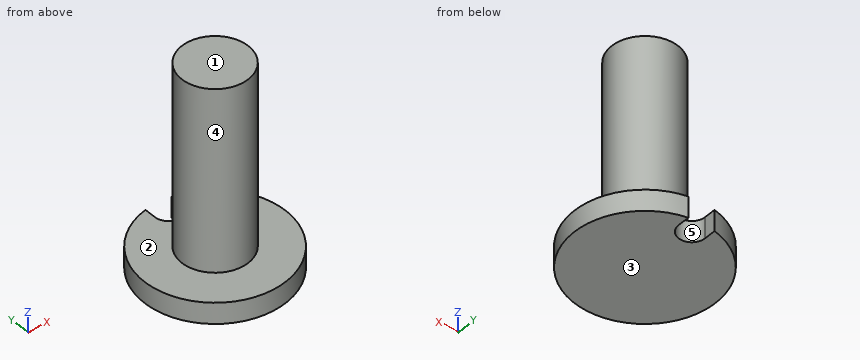
Autodesk Inventor part; units mm, degrees
ref_plane "YZ Plane" through (0, 0, 0) normal (1, 0, 0) x (0, 1, 0)
ref_plane "XZ Plane" through (0, 0, 0) normal (0, 1, 0) x (-1, 0, 0)
ref_plane "XY Plane" through (0, 0, 0) normal (0, 0, 1) x (1, 0, 0)
sketch "Sketch1" plane through (0, 0, 0) normal (0, 0, 1) x (1, 0, 0)
  circle A0 centre (0, 0) radius 8.509
  dimension "d0" = 17.018
extrude "Extrusion1" add sketch "Sketch1" along normal blind 2.54
sketch "Sketch3" plane through (0, 0, 0) normal (0, 0, -1) x (-1, 0, 0)
  line L0 (0, 0) -> (0, 6.9342)
  circle A0 centre (0, 6.9342) radius 1.5875
  line L1 (-1.5875, 6.9342) -> (-1.5875, 8.3596)
  circle A1 centre (0, 0) radius 8.509
  line L2 (1.5875, 6.9342) -> (1.5875, 8.3596)
  dimension "d6" = 6.9342
  dimension "d7" = 3.175
extrude "Extrusion3" cut sketch "Sketch3" against normal through all contours A0 A1 | A0 A1 L2 | A0 L1 A1 picked at (-0.1424, 6.414)
sketch "Sketch2" plane through (0, 0, 2.54) normal (0, 0, 1) x (1, 0, 0)
  circle A0 centre (0, 0) radius 8.509
  circle A1 centre (0, 0) radius 4.0005
  dimension "d3" = 8.001
extrude "Extrusion2" add sketch "Sketch2" along normal blind 21.971 contours A1
properties part number "pulley shaft"
Check sheet for the modelled part. Datum: model origin and axes. Units: mm. Face numbers are marked on the shaded views. A direction names the side the tool comes from. Give positions to 0.01 mm unless a question says otherwise; leave off trailing zeros. Write each loop counter-clockwise with the first axis right and the second up, starting at its lowest first coordinate (ties: lowest second). Pieces come first, ordered by that corner, then holes. Notation, with made-up numbers: (83.25, 64) -> (111.25, 64) arc R10 cw to (111.25, 73) -> close; hole circle Ø5 at (35, -3.75). An arc over 180 degrees is marked (long way). Use one line per item in the form item = value. Start each with the question number.
1. Go/stop test with flat-tipped pins: P1, Ø6, axis at y = 0.5, z = 19.5, coming from the +X side; P2, Ø5, axis at x = 0.5, z = 9.5, coming from the -Y side; P3, Ø4, axis at y = 5, z = 15, coming from the -X side. Record where each tip stops, or that it passes through.
2. Access from +Z, -Z, +X, -X, +Y, -Y to the whole of each face (thin tool, end or side, straight path). Record for the marked faces 1 and 2.
3. Section check D-D (x = -7). Record the cut outline in (y, z), and give its area (3 significant figures).
4. Section check A-A (x = 0). Record the cut outline in (y, z).
5. Thickness scan on line 1 along Z through (x, y) = (6.5, 3.5); line 2 along Y through (x, z) = (-2, 21); line 3 along X through (y, z) = (1.25, 15.75). Record the ranges inside material, lowest first. Write a range as from..to.
6. Section check C-C (z = 8). Record the cut outline in (x, y), and give its area (3 significant figures).
7. Mould release check, pull along X, two halves, no side actions. Record for the marked faces 3, 4 and 5: pulls with the +X half, pulls with the -X half, needs draft (parallel to the pull), parting line crosses it, or undercut.
8. Section check B-B (y = 0). Record the cut outline in (x, z).
Conclusion:
q1.P1 = 4
q1.P2 = -4
q1.P3 = -2.65
q2.face_1 = +Z, +X, -X, +Y, -Y
q2.face_2 = +Z
q3.outline = (-4.84, 0) -> (4.84, 0) -> (4.84, 2.54) -> (-4.84, 2.54) -> close
q3.area = 24.6 mm²
q4.outline = (-8.51, 0) -> (5.35, 0) -> (5.35, 2.54) -> (4, 2.54) -> (4, 24.51) -> (-4, 24.51) -> (-4, 2.54) -> (-8.51, 2.54) -> close
q5.line_1 = 0..2.54
q5.line_2 = -3.46..3.46
q5.line_3 = -3.8..3.8
q6.outline = circle Ø8 at (0, 0)
q6.area = 50.3 mm²
q7.face_3 = needs draft
q7.face_4 = parting line crosses it
q7.face_5 = undercut
q8.outline = (-8.51, 0) -> (8.51, 0) -> (8.51, 2.54) -> (4, 2.54) -> (4, 24.51) -> (-4, 24.51) -> (-4, 2.54) -> (-8.51, 2.54) -> close
